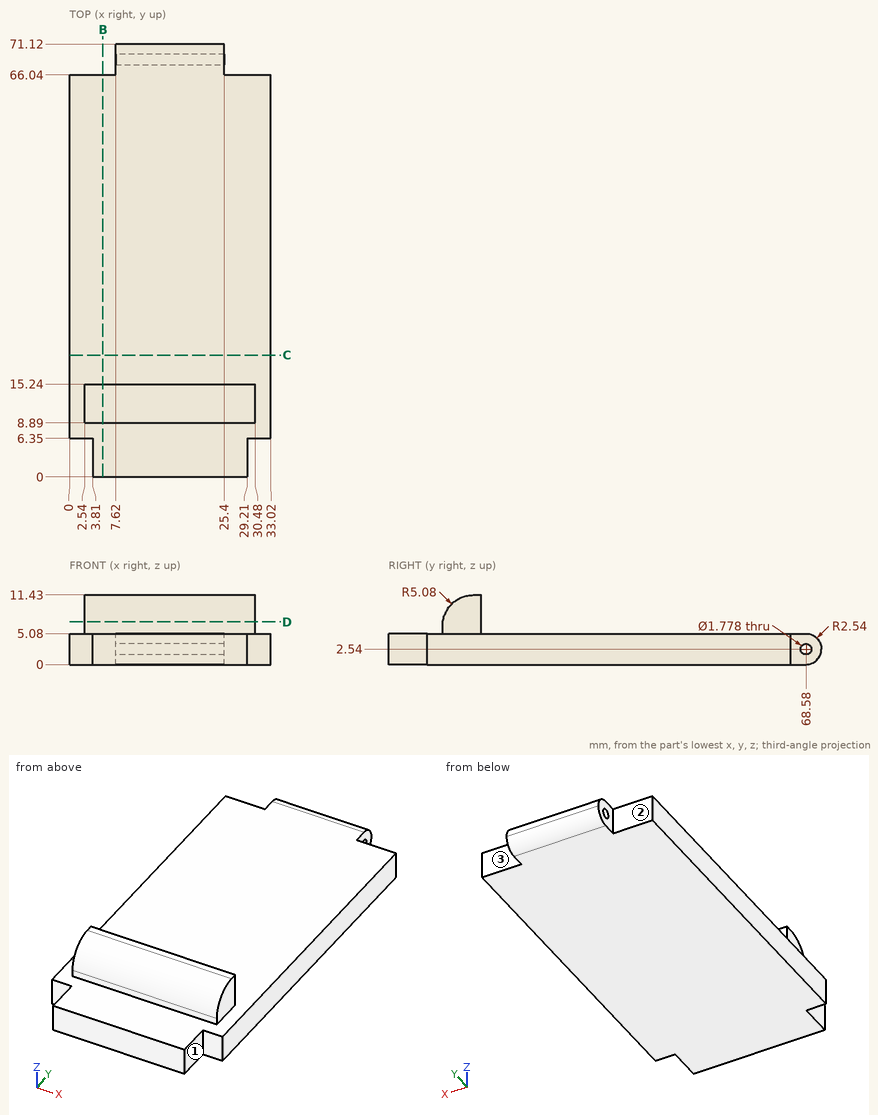
Input: dimensioned drawing with shaded views. Units: mm. Origin: part minimum x, y, z. A direction names the side the tool comes from. Give positions to 0.01 mm unless a question says otherwise; leave off trailing zeros. Order: outer loops, then holes, each group sorted by start corner. A loop starts at its lowest first (then second) coordinate and runs counter-clockwise, first axis right, second up. Notation, with made-up numbers: (1, -4) -> (21, -4) arc R31 ccw to (21, 25) -> close; hole circle Ø3 at (2.25, 22.5). An arc over 180 degrees is marked (long way). Answer as a JSON object with one key per item and string values.
Q1. Material intervals for probe 1 along Z at (x, y) = (12.5, 68.58); probe 2 along Z at (x, y) = (20.5, 6); probe 3 along Y at (x, z) = (24.5, 5.5), sorted ascending.
Entries:
{"probe 1": "z = 0 to 1.65, 3.43 to 5.08", "probe 2": "z = 0 to 5.08", "probe 3": "y = 8.89 to 15.24"}
Q2. Access query for the marked faces 1, 2 and 3. Directions: +Z, -Z, +X, -X, +Y, -Y. A direction counts if a zero-diameter tool reaches every point of the face in a straight line with its end or side. Return the directions, or none.
Entries:
{"face 1": "+Z, -Z, +X, -Y", "face 2": "+Z, -Z, -X, +Y", "face 3": "+Z, -Z, +X, +Y"}
Q3. Section C-C (y = 20). Output: boundary loops of the cut face in (x, z), plus the area to 3 significant figures.
Entries:
{"outline": "(0, 0) -> (33.02, 0) -> (33.02, 5.08) -> (0, 5.08) -> close", "area": "168 mm^2"}
Q4. Section D-D (z = 7). Output: boundary loops of the cut face in (x, y), plus the area to 3 significant figures.
Entries:
{"outline": "(2.54, 8.93) -> (30.48, 8.93) -> (30.48, 15.24) -> (2.54, 15.24) -> close", "area": "176 mm^2"}
Q5. Section B-B (x = 5.5). Output: boundary loops of the cut face in (y, z), plus the area to 3 significant figures.
Entries:
{"outline": "(0, 0) -> (66.04, 0) -> (66.04, 5.08) -> (15.24, 5.08) -> (15.24, 11.43) -> (13.97, 11.43) arc R5.08 ccw to (8.89, 6.35) -> (8.89, 5.08) -> (0, 5.08) -> close", "area": "370 mm^2"}
Q6. First-contact query: pin 1 (1.5 mm diameter, centred on y = 68.5, z = 3.5, fed in from -X); pin 2 (1.1 mm diameter, centred on x = 1.5, z = 1.5, fed in from -Y); pin 3 (0.6 mm diameter, centred on x = 16, z = 6, fed in from -Y); pin 4 (4 mm diameter, centred on x = 30.5, z = 2.5, fed in from -Y). Flat tips, straight axial feed; report the tip coordinate or a pass-through.
Entries:
{"pin 1": "stops at x = 7.62", "pin 2": "stops at y = 6.35", "pin 3": "stops at y = 8.89", "pin 4": "stops at y = 0"}
